from build123d import *

# Parameters (mm, degrees)
SKETCH1_R           = 5
BOSS_EXTRUDE1_DEPTH = 10
CUT_EXTRUDE1_DEPTH  = 320.43525409


with BuildPart() as part:
    # Sketch1 → Boss-Extrude1 (new body)
    with BuildSketch(Plane.XY):
        Polygon((300, -109.265189129), (300, -92.815809214), (194.210465663, 70.734810871), (-194.210465663, 70.734810871), (-300, -92.815809214), (-300, -109.265189129), align=None)
        with Locations((-187.3, 58.034810871)):
            Circle(SKETCH1_R, mode=Mode.SUBTRACT)
        with Locations((-287.3, -96.565189129)):
            Circle(SKETCH1_R, mode=Mode.SUBTRACT)
        with Locations(Location((287.3, -96.565189129, 0), (0, 0, 180))):
            Circle(SKETCH1_R, mode=Mode.SUBTRACT)
        with Locations(Location((187.3, 58.034810871, 0), (0, 0, 180))):
            Circle(SKETCH1_R, mode=Mode.SUBTRACT)
    extrude(amount=BOSS_EXTRUDE1_DEPTH)

    # Sketch2 → Cut-Extrude1 (cut, through all)
    with BuildSketch(Plane.XY.offset(10)):
        Polygon((180.863413893, 36.132549959), (261.974499978, -89.265189129), (-259.820043515, -89.265189129), align=None)
        Polygon((-250.097346147, -70.903109306), (177.373034147, 50.734810871), (-171.418225722, 50.734810871), align=None)
    extrude(amount=-CUT_EXTRUDE1_DEPTH, mode=Mode.SUBTRACT)


solid = part.part
Source: CAD feature listing. Evaluate the final solid. Frame: model axes, mm. A direction names the side the tool comes from. Give positions to 0.01 mm unless a question says otherwise; leave off trailing zeros. Loops run counter-clockwise (first coordinate to the right, second up) from the corner with the lowest first, then second, coordinate; pieces in that order, holes last. Notation, with made-up numbers: (21, 73) -> (79, 73) arc R27 cw to (79, 90) -> close; hole circle Ø3 at (-17, 85.25). An arc over 180 degrees is marked (long way). Use a Markdown table: item, result. Add a question column.
1) Section query C-C, the plane z = 7.25. Return the cut outline in (x, y), then the cut area to 3 significant figures.
2) Section query B-B, the plane x = 160.5. Return the cut outline in (y, z).
3) Pull-direction query (X, two-part tool) for faces 3 (the face through (-4, -109.265, 5)), 4 (the face through (5, 50.735, 5)), 5 (the face through (300, -101, 5)), 6 (the face through (-300, -101, 5)); classes: +X half, -X half, draft (parallel to the pull), parting line (faces both ways), or undercut.
4) Line query: line 1 along Y through (x, z) = (187.3, 7); line 2 along Y through (x, z) = (5, 8.25); line 3 along Y through (x, z) = (-187.3, 5.5). Output: solid intervals per line, ascending. Write a range as [from, to].
5) First-contact query: pin 1 (1 mm diameter, centred on y = -88, z = 5, fed in from -X); pin 2 (4 mm diameter, centred on y = 23, z = 1.5, fed in from +X); pin 3 (1.5 mm diameter, centred on y = 13, z = 1.5, fed in from +X). Flat tips, straight axial feed; report the tip coordinate or a pass-through.
6) Section query A-A, the plane y = -55. Return the cut outline in (x, z), then the cut area to 3 significant figures.
7) Reachability of faces 1 (the face through (-210.207, -9.233, 5.07)), 2 (the face through (-24, -19, 10)) from +Z, -Z, +X, -X, +Y, -Y: full face, straight path, thin tool, end or side. Return the list, or none.
Numbers:
| question | item | result |
|---|---|---|
| 1 | outline | (-300, -109.27) -> (300, -109.27) -> (300, -92.82) -> (194.21, 70.73) -> (-194.21, 70.73) -> (-300, -92.82) -> close; hole circle Ø10 at (-287.3, -96.57); hole (-259.82, -89.27) -> (261.97, -89.27) -> (180.86, 36.13) -> close; hole (-250.1, -70.9) -> (177.37, 50.73) -> (-171.42, 50.73) -> close; hole circle Ø10 at (-187.3, 58.03); hole circle Ø10 at (187.3, 58.03); hole circle Ø10 at (287.3, -96.57) |
| 1 | area | 36,500 mm2 |
| 2 | outline | (-109.27, 0) -> (-89.27, 0) -> (-89.27, 10) -> (-109.27, 10) -> close; (30.34, 0) -> (45.93, 0) -> (45.93, 10) -> (30.34, 10) -> close; (50.73, 0) -> (70.73, 0) -> (70.73, 10) -> (50.73, 10) -> close |
| 3 | face 3 | draft |
| 3 | face 4 | undercut |
| 3 | face 5 | +X half |
| 3 | face 6 | -X half |
| 4 | line 1 | y = [-109.27, -89.27], [26.18, 53.03], [63.03, 70.73] |
| 4 | line 2 | y = [-109.27, -89.27], [-13.91, 1.69], [50.73, 70.73] |
| 4 | line 3 | y = [-109.27, -89.27], [-68.63, -53.03], [26.18, 53.03], [63.03, 70.73] |
| 5 | pin 1 | stops at x = -297.21 |
| 5 | pin 2 | stops at x = 226.38 |
| 5 | pin 3 | stops at x = 232.04 |
| 6 | outline | (-275.54, 0) -> (-239.81, 0) -> (-239.81, 10) -> (-275.54, 10) -> close; (-194.21, 0) -> (-139.4, 0) -> (-139.4, 10) -> (-194.21, 10) -> close; (239.81, 0) -> (275.54, 0) -> (275.54, 10) -> (239.81, 10) -> close |
| 6 | area | 1,260 mm2 |
| 7 | face 1 | +Z, -Z |
| 7 | face 2 | +Z, +X, -X, +Y, -Y |
